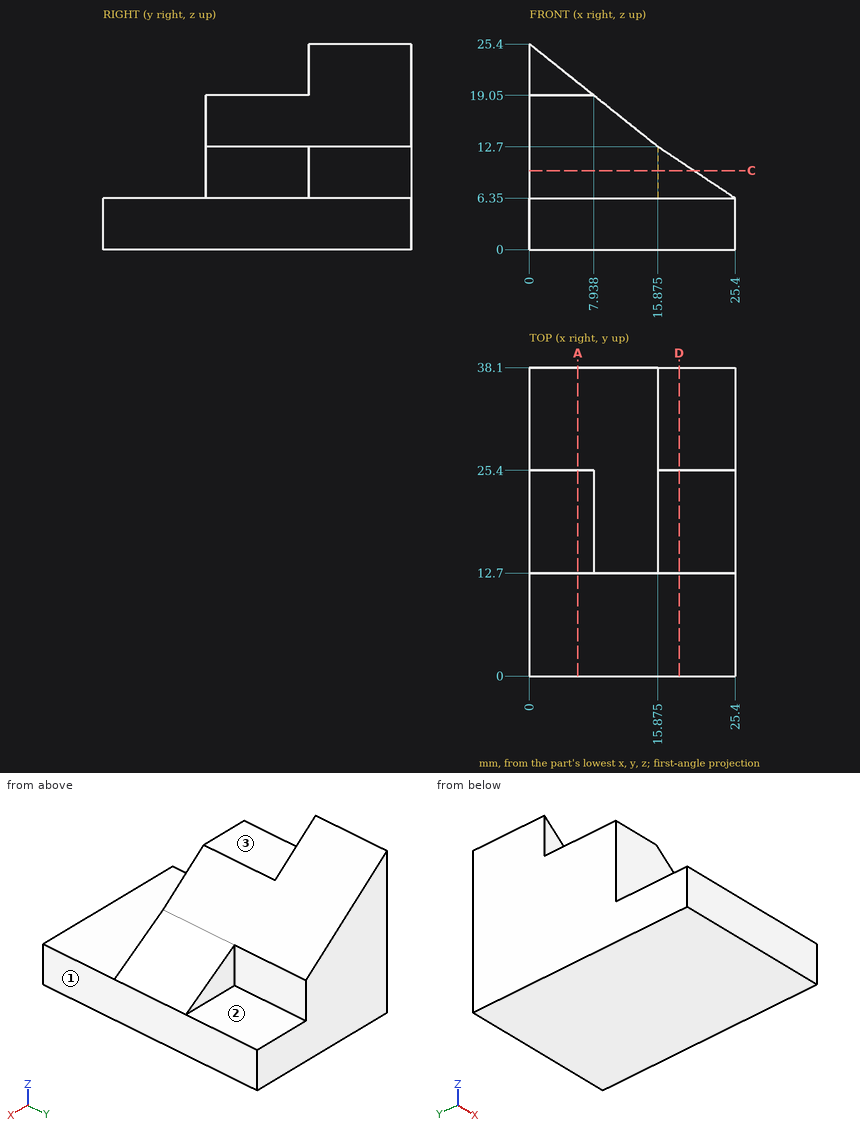
Input: dimensioned drawing with shaded views. Units: mm. Origin: part minimum x, y, z. A direction names the side the tool comes from. Round coordinates to 2 decimals unless told otherwise and drop trailing zeros. Order: outer loops, then holes, each group sorted by start corner. A loop starts at its lowest first (then second) coordinate and runs counter-clockwise, first axis right, second up. Notation, with made-up numbers: (68.25, 22.25) - (80.25, 22.25) arc R9 cw to (80.25, 30.25) - close; hole circle Ø4 at (80, -1). An arc over 180 degrees is marked (long way). Write item = value, one per line. Start each with the question number.
Q1. Access query for the marked faces 1, 2 and 3. Directions: +Z, -Z, +X, -X, +Y, -Y. A direction counts if a zero-diameter tool reaches every point of the face in a straight line with its end or side. Return the directions, or none.
Q2. Cut plane A-A on x = 6. Return the cut outline in (y, z).
Q3. Cut plane D-D on x = 18.5. Return the cut outline in (y, z).
Q4. Ray query, line 1 (X direction, y = 29.5, z = 7.75) (1 decimal); line 2 (Y direction, x = 9, z = 15.25); line 3 (Z direction, x = 13, y = 12). Return the intervals inside material, ascending. Write a range as from..to.
Q5. Pin query (flat end, axial travel): pin 1 (6.5 mm diameter, centred on x = 10.5, z = 13.5, fed in from -Y); pin 2 (10 mm diameter, centred on x = 11, y = 24, fed in from +Z); pin 3 (10.5 mm diameter, centred on x = 21, y = 30, fed in from +Z); pin 4 (2 mm diameter, centred on y = 5.5, z = 8.5, fed in from +X). Return the tip coordinate at first contact, or that it passes through.
Q6. Cut plane C-C on z = 9.75. Return the cut outline in (x, y) (1 decimal).
Outcome:
q1.face_1 = +Z, -Z, +X, +Y, -Y
q1.face_2 = +Z, +X, +Y
q1.face_3 = +Z, +X, -X, -Y
q2.outline = (0, 0) - (38.1, 0) - (38.1, 20.6) - (25.4, 20.6) - (25.4, 19.05) - (12.7, 19.05) - (12.7, 6.35) - (0, 6.35) - close
q3.outline = (0, 0) - (38.1, 0) - (38.1, 6.35) - (25.4, 6.35) - (25.4, 10.95) - (12.7, 10.95) - (12.7, 6.35) - (0, 6.35) - close
q4.line_1 = 0..15.9
q4.line_2 = 12.7..38.1
q4.line_3 = 0..6.35
q5.pin_1 = 12.7
q5.pin_2 = 20.44
q5.pin_3 = 12.8
q5.pin_4 = through
q6.outline = (0, 12.7) - (20.3, 12.7) - (20.3, 25.4) - (15.9, 25.4) - (15.9, 38.1) - (0, 38.1) - close
